```python
from build123d import *

# Parameters (mm, degrees)
IZIM1_R                      = 150
Y_KSEKLIK_EKSTR_ZYON1_DEPTH  = 70
Y_KSEKLIK_EKSTR_ZYON14_DEPTH = 5
Y_KSEKLIK_EKSTR_ZYON16_DEPTH = 17.5
KES_EKSTR_ZYON1_DEPTH        = 27.5
KES_EKSTR_ZYON3_DEPTH        = 7.5
Y_KSEKLIK_EKSTR_ZYON17_DEPTH = 6
DAIRESEL_KAPLAMA1_COUNT      = 4
DAIRESEL_KAPLAMA2_COUNT      = 4
RADYUS1_R                    = 10
IZIM19_R                     = 2
KES_EKSTR_ZYON5_DEPTH        = 10
IZIM22_R                     = 140
Y_KSEKLIK_EKSTR_ZYON18_DEPTH = 1
KES_EKSTR_ZYON8_DEPTH        = 11
KES_EKSTR_ZYON8_DEPTH_BACK   = 31
IZIM18_W                     = 42
IZIM18_H                     = 42


with BuildPart() as part:
    # Çizim1 → Yükseklik-Ekstrüzyon1 (new body)
    with BuildSketch(Plane(origin=(0, 0, 0), x_dir=(1, 0, 0), z_dir=(0, 1, 0))):
        with Locations(Location((0, 0, 0), (0, 0, 270))):
            Circle(IZIM1_R)
    extrude(amount=Y_KSEKLIK_EKSTR_ZYON1_DEPTH)

    # Çizim2 → Yükseklik-Ekstrüzyon14 (add)
    with BuildSketch(Plane(origin=(0, 0, 0), x_dir=(1, 0, 0), z_dir=(0, 1, 0))):
        with BuildLine():
            Line((-19.938381567, 146.7204745), (-19.959218349, 172.993465408))
            Line((-19.959218349, 172.993465408), (19.834593255, 172.993465408))
            Line((19.834593255, 172.993465408), (19.793688749, 146.733102083))
            add(Edge.make_bspline(
                [(-19.938381567, 146.7204745), (-6.821574105, 149.387431492), (6.677589472, 149.400040821), (19.793688749, 146.733102083)],
                knots=[0, 0, 0, 0, 0.935808431, 0.935808431, 0.935808431, 0.935808431], degree=3))
        make_face()
    y_kseklik_ekstr_zyon14 = extrude(amount=Y_KSEKLIK_EKSTR_ZYON14_DEPTH)

    # Çizim11 → Yükseklik-Ekstrüzyon16 (add)
    with BuildSketch(Plane(origin=(0, 5, 0), x_dir=(1, 0, 0), z_dir=(0, 1, 0))):
        Polygon((-19.957686049, 171.061396107), (-17.341172439, 171.061396107), (-17.341172439, 146.643122555), (-19.949304151, 146.643122555), align=None)
        Polygon((17.194554667, 146.643122555), (19.802686379, 146.643122555), (19.811068277, 171.061396107), (17.194554667, 171.061396107), align=None)
    y_kseklik_ekstr_zyon16 = extrude(amount=Y_KSEKLIK_EKSTR_ZYON16_DEPTH)

    # Çizim12 → Kes-Ekstrüzyon1 (cut, symmetric)
    with BuildSketch(Plane(origin=(0, 0, 0), x_dir=(0, 0, -1), z_dir=(1, 0, 0))):
        Polygon((155.535554898, 23.200577764), (171.374705499, 7.361427163), (171.374705499, 23.200577764), align=None)
    kes_ekstr_zyon1 = extrude(amount=KES_EKSTR_ZYON1_DEPTH, both=True, mode=Mode.SUBTRACT)

    # Çizim13 → Kes-Ekstrüzyon3 (cut)
    with BuildSketch(Plane(origin=(0, 0, 0), x_dir=(1, 0, 0), z_dir=(0, 1, 0))):
        Polygon((-19.957686049, 171.061396107), (-17.341172439, 173.196821818), (-20.112409128, 173.196821818), (-20.112409128, 171.061396107), align=None)
        Polygon((20.112409128, 173.196821818), (20.112409128, 171.061396107), (19.957686049, 171.061396107), (17.341172439, 173.196821818), align=None)
    kes_ekstr_zyon3 = extrude(amount=KES_EKSTR_ZYON3_DEPTH, mode=Mode.SUBTRACT)

    # Çizim17 → Yükseklik-Ekstrüzyon17 (add)
    with BuildSketch(Plane(origin=(0, 0, 0), x_dir=(1, 0, 0), z_dir=(0, 1, 0))):
        Polygon((11.703099503, 121.823652722), (9.703099523, 121.82337545), (8.703339657, 120.091186024), (9.703579771, 118.359273869), (11.703579752, 118.35955114), (12.703339618, 120.091740567), align=None)
        Polygon((-9.703579771, 118.359273869), (-11.703579752, 118.35955114), (-12.703339618, 120.091740567), (-11.703099503, 121.823652722), (-9.703099523, 121.82337545), (-8.703339657, 120.091186024), align=None)
    y_kseklik_ekstr_zyon17 = extrude(amount=Y_KSEKLIK_EKSTR_ZYON17_DEPTH)

    # Dairesel Kaplama1: Yükseklik-Ekstrüzyon14, Yükseklik-Ekstrüzyon16, Kes-Ekstrüzyon3, Yükseklik-Ekstrüzyon17 ×4 about axis
    dairesel_kaplama1_axis = Axis((0, 0, 0), (0, 1, 0))
    add([y_kseklik_ekstr_zyon14.rotate(dairesel_kaplama1_axis, i * 360 / DAIRESEL_KAPLAMA1_COUNT) for i in range(1, DAIRESEL_KAPLAMA1_COUNT)])
    add([y_kseklik_ekstr_zyon16.rotate(dairesel_kaplama1_axis, i * 360 / DAIRESEL_KAPLAMA1_COUNT) for i in range(1, DAIRESEL_KAPLAMA1_COUNT)])
    add([kes_ekstr_zyon3.rotate(dairesel_kaplama1_axis, i * 360 / DAIRESEL_KAPLAMA1_COUNT) for i in range(1, DAIRESEL_KAPLAMA1_COUNT)], mode=Mode.SUBTRACT)
    add([y_kseklik_ekstr_zyon17.rotate(dairesel_kaplama1_axis, i * 360 / DAIRESEL_KAPLAMA1_COUNT) for i in range(1, DAIRESEL_KAPLAMA1_COUNT)])

    # Dairesel Kaplama2: Kes-Ekstrüzyon1 ×4 about axis
    dairesel_kaplama2_axis = Axis((0, 0, 0), (0, 1, 0))
    for i in range(1, DAIRESEL_KAPLAMA2_COUNT):
        add(kes_ekstr_zyon1.rotate(dairesel_kaplama2_axis, i * 360 / DAIRESEL_KAPLAMA2_COUNT), mode=Mode.SUBTRACT)

    # Radyus1
    radyus1_edges = [part.edges().sort_by_distance(p)[0] for p in [
        (0, 70, -150),
    ]]
    fillet(radyus1_edges, radius=RADYUS1_R)

    # Çizim19 → Kes-Ekstrüzyon5 (cut)
    with BuildSketch(Plane(origin=(0, 5, 0), x_dir=(1, 0, 0), z_dir=(0, 1, 0))):
        with Locations(Location((-12.590175798, 168.65903489, 0), (0, 0, 270))):
            Circle(IZIM19_R)
        with Locations(Location((12.590175798, 168.65903489, 0), (0, 0, 270))):
            Circle(IZIM19_R)
        with Locations(Location((168.65903489, 12.590175798, 0), (0, 0, 270))):
            Circle(IZIM19_R)
        with Locations(Location((168.65903489, -12.590175798, 0), (0, 0, 270))):
            Circle(IZIM19_R)
        with Locations(Location((12.590175798, -168.65903489, 0), (0, 0, 270))):
            Circle(IZIM19_R)
        with Locations(Location((-12.590175798, -168.65903489, 0), (0, 0, 270))):
            Circle(IZIM19_R)
        with Locations(Location((-168.65903489, -12.590175798, 0), (0, 0, 270))):
            Circle(IZIM19_R)
        with Locations(Location((-168.65903489, 12.590175798, 0), (0, 0, 270))):
            Circle(IZIM19_R)
    extrude(amount=-KES_EKSTR_ZYON5_DEPTH, mode=Mode.SUBTRACT)

    # Çizim22 → Yükseklik-Ekstrüzyon18 (add)
    with BuildSketch(Plane(origin=(0, 70, 0), x_dir=(1, 0, 0), z_dir=(0, 1, 0))):
        Circle(IZIM22_R)
    extrude(amount=-Y_KSEKLIK_EKSTR_ZYON18_DEPTH)

    # Çizim18 → Kes-Ekstrüzyon8 (cut, two sides: drawn at the far end of the back side and taken through both)
    with BuildSketch(Plane(origin=(0, 70, 0), x_dir=(1, 0, 0), z_dir=(0, 1, 0)).offset(-KES_EKSTR_ZYON8_DEPTH_BACK)):
        Rectangle(IZIM18_W, IZIM18_H)
    extrude(amount=KES_EKSTR_ZYON8_DEPTH + KES_EKSTR_ZYON8_DEPTH_BACK, mode=Mode.SUBTRACT)


solid = part.part
```
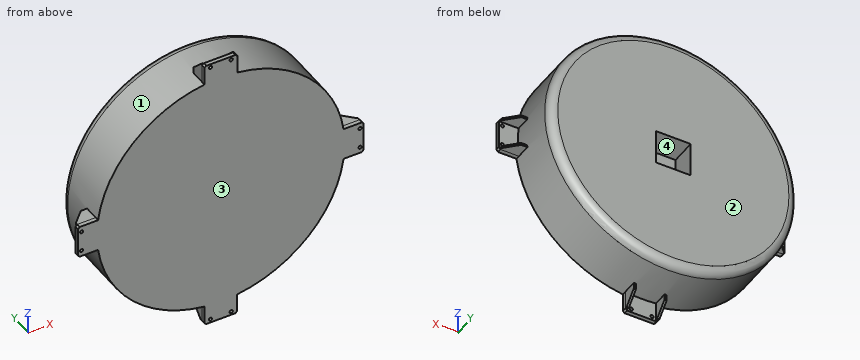
Check sheet for the modelled part. Datum: model origin and axes. Units: mm. Face numbers are marked on the shaded views. A direction names the side the tool comes from. Round coordinates to 2 decimals unless told otherwise and drop trailing zeros. Order: outer loops, then holes, each group sorted by start corner. A loop starts at its lowest first (then second) coordinate and runs counter-clockwise, first axis right, second up. Notation, with made-up numbers: (8.5, 36) -> (51.5, 36) arc R17 ccw to (51.5, 57) -> close; hole circle Ø3 at (85.5, 23). An arc over 180 degrees is marked (long way). One line per item, written item: value. Start each with the question number.
Q1. Set-up check for the marked faces 1 and 2: record each of +Z, -Z, +X, -X, +Y, -Y from which the full face is reachable in a straight line by a thin tool's end or side.
Q2. Thickness scan on line 1 (Z direction, x = 155.5, y = 18); line 2 (Y direction, x = -129.5, z = -54); line 3 (X direction, y = 12, z = 0). Record the ranges inside material, lowest first.
Q3. Cross-section at D-D (y = 27.5). Record the boundary of the cut face in (x, z).
Q4. Cross-section at C-C (y = 52.5). Record the boundary of the cut face in (x, z).
Q5. Gauge pin test, flat ends, axial feed: pin 1 Ø2 at (x, y) = (18.5, 6.5) entering from +Z; pin 2 Ø12.5 at (x, z) = (-2, -1.5) entering from +Y; pin 3 Ø0.8 at (x, z) = (-151.5, -18) entering from +Y; pin 4 Ø4.5 at (x, z) = (12.59, -168.66) entering from -Y. Record the tip position at first contact, or that the pin passes through.
Q6. Cross-section at B-B (x = 0). Record the boundary of the cut face in (y, z).
Q7. Mould release check, pull along Z, two halves, no side actions. Record for the marked faces 3 and 4: pulls with the +Z half, pulls with the -Z half, needs draft (parallel to the pull), parting line crosses it, or undercut.
Q8. Cross-section at A-A (z = 0). Record the boundary of the cut face in (x, y), and give its area (3 significant figures).
Completed:
1. face 1: +Y
1. face 2: +Z, -Z, +X, -X, +Y
2. line 1: z = -19.95 to -17.34, 17.19 to 19.81
2. line 2: y = 0 to 70
2. line 3: x = -150 to 150
3. outline: circle Ø300 at (0, 0)
4. outline: circle Ø300 at (0, 0); hole (-21, -21) -> (21, -21) -> (21, 21) -> (-21, 21) -> close
5. pin 1: stops at z = 171.06
5. pin 2: stops at y = 39
5. pin 3: stops at y = 22.5
5. pin 4: stops at y = 0
6. outline: (0, -172.99) -> (5, -172.99) -> (5, -150) -> (60, -150) arc R10 ccw to (70, -140) -> (70, -21) -> (39, -21) -> (39, 21) -> (70, 21) -> (70, 140) arc R10 ccw to (60, 150) -> (5, 150) -> (5, 172.99) -> (0, 172.99) -> close
7. face 3: needs draft
7. face 4: undercut
8. outline: (-172.99, 0) -> (172.99, 0) -> (172.99, 5) -> (150, 5) -> (150, 60) arc R10 ccw to (140, 70) -> (21, 70) -> (21, 39) -> (-21, 39) -> (-21, 70) -> (-140, 70) arc R10 ccw to (-150, 60) -> (-150, 5) -> (-172.99, 5) -> close
8. area: 19,900 mm²
